from build123d import *

# Parameters (mm, degrees)
SKETCH_1_W      = 10.6
SKETCH_1_H      = 10.6
EXTRUDE_1_DEPTH = 1000


with BuildPart() as part:
    # Эскиз1 → Бобышка-Вытянуть1 (new body)
    with BuildSketch(Plane.XY):
        Polygon((-20, 7.15), (-20, 20), (-7.15, 20), (-4.2, 20), (-4.2, 18.5), (-7.15, 18.5), (-7.15, 8.15), (-6.15, 7.15), (-0.7, 7.15), (0, 6.45), (0.7, 7.15), (6.15, 7.15), (7.15, 8.15), (7.15, 18.5), (4.2, 18.5), (4.2, 20), (7.15, 20), (20, 20), (20, 7.15), (20, 4.2), (18.5, 4.2), (18.5, 7.15), (8.15, 7.15), (7.15, 6.15), (7.15, 0.7), (6.45, 0), (7.15, -0.7), (7.15, -6.15), (8.15, -7.15), (18.5, -7.15), (18.5, -4.2), (20, -4.2), (20, -7.15), (20, -20), (7.15, -20), (4.2, -20), (4.2, -18.5), (7.15, -18.5), (7.15, -8.15), (6.15, -7.15), (0.7, -7.15), (0, -6.45), (-0.7, -7.15), (-6.15, -7.15), (-7.15, -8.15), (-7.15, -18.5), (-4.2, -18.5), (-4.2, -20), (-7.15, -20), (-20, -20), (-20, -7.15), (-20, -4.2), (-18.5, -4.2), (-18.5, -7.15), (-8.15, -7.15), (-7.15, -6.15), (-7.15, -0.7), (-6.45, 0), (-7.15, 0.7), (-7.15, 6.15), (-8.15, 7.15), (-18.5, 7.15), (-18.5, 4.2), (-20, 4.2), align=None)
        with Locations((13.6, 13.6)):
            Rectangle(SKETCH_1_W, SKETCH_1_H, mode=Mode.SUBTRACT)
        with Locations((-13.6, 13.6)):
            Rectangle(SKETCH_1_W, SKETCH_1_H, mode=Mode.SUBTRACT)
        with Locations((13.6, -13.6)):
            Rectangle(SKETCH_1_W, SKETCH_1_H, mode=Mode.SUBTRACT)
        with Locations((-13.6, -13.6)):
            Rectangle(SKETCH_1_W, SKETCH_1_H, mode=Mode.SUBTRACT)
        with BuildLine():
            Line((4.242640687, 5.656854249), (2.937238153, 4.351451715))
            ThreePointArc((2.937238153, 4.351451715), (0, 5.25), (-2.937238153, 4.351451715))
            Line((-2.937238153, 4.351451715), (-4.242640687, 5.656854249))
            ThreePointArc((-4.242640687, 5.656854249), (-5.656854249, 5.656854249), (-5.656854249, 4.242640687))
            Line((-5.656854249, 4.242640687), (-4.351451715, 2.937238153))
            ThreePointArc((-4.351451715, 2.937238153), (-5.25, 0), (-4.351451715, -2.937238153))
            Line((-4.351451715, -2.937238153), (-5.656854249, -4.242640687))
            ThreePointArc((-5.656854249, -4.242640687), (-5.656854249, -5.656854249), (-4.242640687, -5.656854249))
            Line((-4.242640687, -5.656854249), (-2.937238153, -4.351451715))
            ThreePointArc((-2.937238153, -4.351451715), (0, -5.25), (2.937238153, -4.351451715))
            Line((2.937238153, -4.351451715), (4.242640687, -5.656854249))
            ThreePointArc((4.242640687, -5.656854249), (5.656854249, -5.656854249), (5.656854249, -4.242640687))
            Line((5.656854249, -4.242640687), (4.351451715, -2.937238153))
            ThreePointArc((4.351451715, -2.937238153), (5.25, 0), (4.351451715, 2.937238153))
            Line((4.351451715, 2.937238153), (5.656854249, 4.242640687))
            ThreePointArc((5.656854249, 4.242640687), (5.656854249, 5.656854249), (4.242640687, 5.656854249))
        make_face(mode=Mode.SUBTRACT)
    extrude(amount=EXTRUDE_1_DEPTH)


solid = part.part
Can you work these out from the model? Positions are in its coordinate system, mm. Give positions to 0.01 mm unless a question says otherwise; leave off trailing zeros. Use one line per item in the form item = value. Start each with the question number.
Item 1: Will these pins go through, and if not, where does the flat tip stop? pin 1 Ø5 at (x, y) = (-14, 2.5) entering from -Z; pin 2 Ø1.6 at (x, z) = (-2.5, 405) entering from +Y.
Item 2: If we section it at A-A (z = 693.5): State how many separate pieces and enclosed holes the cut face has, then the cut area to 3 significant figures.
Item 3: If I drill on line 1 along X through (y, z) = (-9.5, 762); line 2 along X through (y, z) = (-4, 782), over which ranges is the centre line in solid material (lowest first)?
Outcome:
q1.pin_1 = through
q1.pin_2 = 7.15
q2.separate_pieces = 1
q2.enclosed_holes = 5
q2.area = 346 mm2
q3.line_1 = -20 to -18.9, -8.3 to -7.15, 7.15 to 8.3, 18.9 to 20
q3.line_2 = -7.15 to -5.41, 5.41 to 7.15
